Part model, mm, in its own coordinate system. A direction names the side the tool comes from. Round coordinates to 2 decimals unless told otherwise and drop trailing zeros. Order: outer loops, then holes, each group sorted by start corner. A loop starts at its lowest first (then second) coordinate and runs counter-clockwise, first axis right, second up. Notation, with made-up numbers: (45.5, 30.25) -> (96.5, 30.25) arc R19 cw to (96.5, 52.25) -> close; hole circle Ø5 at (10.25, 82). An arc over 180 degrees is marked (long way). Answer as a JSON object with one key per item and string values. Group by question number.
```python
from build123d import *

# Parameters (mm, degrees)
F1_DEPTH = 76.2
F3_DEPTH = 25.4
F4_DEPTH = 25.4
F5_DEPTH = 38.1
F6_DEPTH = 38.1
F7_DEPTH = 38.1
F8_DEPTH = 38.1
F9_DEPTH = 38.1


with BuildPart() as f1:
    # F0 (on Front) → F1 (new body)
    with BuildSketch(Plane.XZ):
        Polygon((22.4569932461, 74.4162100717), (-18.4116067539, 74.4162100717), (-26.8437221389, 1.1637246492), (13.1697589532, 0), align=None)
    extrude(amount=F1_DEPTH)

    # F2 (on Front) + F1_face (on face) → F3 (cut)
    with BuildSketch(Plane.XZ):
        Polygon((12.081772089, 66.8269023299), (-11.4912800491, 66.8269023299), (-18.7445282936, 10.2515770122), (4.1031986475, 10.2515770122), align=None)
    with BuildSketch(Plane(origin=(-2.3405186652, -76.2, 37.6069334432), x_dir=(1, 0, 0), z_dir=(0, -1, 0))):
        Polygon((-24.5032034737, -36.443208794), (15.5102776183, -37.6069334432), (24.7975119113, 36.8092766285), (-16.0710880887, 36.8092766285), align=None)
    extrude(amount=-F3_DEPTH, mode=Mode.SUBTRACT)

    # F2 (on Front) + F3_face (on face) → F4 (cut)
    with BuildSketch(Plane.XZ):
        Polygon((12.081772089, 66.8269023299), (-11.4912800491, 66.8269023299), (-18.7445282936, 10.2515770122), (4.1031986475, 10.2515770122), align=None)
    with BuildSketch(Plane(origin=(-2.3405186652, -50.8, 37.6069334432), x_dir=(1, 0, 0), z_dir=(0, -1, 0))):
        Polygon((-16.0710880887, 36.8092766285), (-24.5032034737, -36.443208794), (15.5102776183, -37.6069334432), (24.7975119113, 36.8092766285), align=None)
    extrude(amount=-F4_DEPTH, mode=Mode.SUBTRACT)

    # F2 (on Front) → F5 (cut, symmetric)
    with BuildSketch(Plane.XZ):
        Polygon((12.081772089, 66.8269023299), (-11.4912800491, 66.8269023299), (-18.7445282936, 10.2515770122), (4.1031986475, 10.2515770122), align=None)
    extrude(amount=F5_DEPTH, both=True, mode=Mode.SUBTRACT)

    # F2 (on Front) → F6 (join, symmetric)
    with BuildSketch(Plane.XZ):
        Polygon((12.081772089, 66.8269023299), (-11.4912800491, 66.8269023299), (-18.7445282936, 10.2515770122), (4.1031986475, 10.2515770122), align=None)
    extrude(amount=F6_DEPTH, both=True)

    # F7 (cut, symmetric): a face of the model
    f7_faces = [f1.faces().sort_by_distance(p)[0] for p in [
        (-3.4928762861, -38.1, 38.6865713538),
    ]]
    extrude(f7_faces, amount=F7_DEPTH, both=True, mode=Mode.SUBTRACT)

    # F8 (cut, symmetric): a face of the model
    f8_faces = [f1.faces().sort_by_distance(p)[0] for p in [
        (-3.4928762861, 38.1, 38.6865713538),
    ]]
    extrude(f8_faces, amount=F8_DEPTH, both=True, mode=Mode.SUBTRACT)

    # F2 (on Front) → F9 (cut, symmetric)
    with BuildSketch(Plane.XZ):
        Polygon((12.081772089, 66.8269023299), (-11.4912800491, 66.8269023299), (-18.7445282936, 10.2515770122), (4.1031986475, 10.2515770122), align=None)
    extrude(amount=F9_DEPTH, both=True, mode=Mode.SUBTRACT)


solid = f1.part
```
Q1. Band-saw the part on A-A (x = 10.5). List the corners of the cut face in (y, z).
Q2. Band-saw the part on D-D (x = -21). List the corners of the cut face in (y, z), plus the area to 3 significant figures.
Q3. Two-plate mould, pull along X, no slides. Class faces 3 (the flat face through (17.75, -12.52, 36.69)), 4 (the flat face through (8.4, 0, 37.7)), 5 (the flat face through (8.037, -12.878, 38.143)), 6 (the flat face through (-22.57, -12.52, 38.3)): +X half, -X half, draft (parallel to the pull), parting line (faces both ways), or undercut.
Q4. Band-saw the part on B-B (z = 26.5). List the corners of the cut face in (x, y).
Q5. Band-saw the part on C-C (y = -10.5). List the corners of the cut face in (x, z).
Q6. Wall check: line 1 (Z direction, x = 0, y = -16.5); line 2 (Z direction, x = -4, y = -3); line 3 (X direction, y = -20.25, z = 48.5). Give the ranges that are in metal, low to high. Write a range as [from, to].
Q7. Which spindle directions (+Z, -Z, +X, -X, +Y, -Y) get a long thin tool onto all of the face, cutting with end or side? Do faces 1 (the flat face through (8.4, -25.4, 37.7)), 2 (the flat face through (-7, -13, 10.252)). Say none if no direction does.
Q8. Drop flat-ended pins along their axis: pin 1 Ø12 at (x, y) = (-5, -18) entering from -Z; pin 2 Ø2 at (y, z) = (-2.5, 36.5) entering from -X; pin 3 Ø4 at (x, z) = (-20, 11.5) entering from +Y; pin 4 Ø4 at (y, z) = (-16, 38.5) entering from -X. Give the stop position or say it passes through.
Completed:
{
 "1": {"outline": "(-25.4, 0.08) -> (0, 0.08) -> (0, 55.61) -> (-25.4, 55.61) -> close; (-25.4, 66.83) -> (0, 66.83) -> (0, 74.42) -> (-25.4, 74.42) -> close"},
 "2": {"outline": "(-25.4, 0.99) -> (0, 0.99) -> (0, 51.93) -> (-25.4, 51.93) -> close", "area": "1,290 mm2"},
 "3": {"face 3": "+X half", "face 4": "draft", "face 5": "undercut", "face 6": "-X half"},
 "4": {"outline": "(-23.93, -25.4) -> (-16.66, -25.4) -> (-16.66, 0) -> (-23.93, 0) -> close; (6.39, -25.4) -> (16.48, -25.4) -> (16.48, 0) -> (6.39, 0) -> close"},
 "5": {"outline": "(-26.84, 1.16) -> (13.17, 0) -> (22.46, 74.42) -> (-18.41, 74.42) -> close; hole (-18.74, 10.25) -> (4.1, 10.25) -> (12.08, 66.83) -> (-11.49, 66.83) -> close"},
 "6": {"line 1": "[0.38, 10.25], [66.83, 74.42]", "line 2": "[0.5, 10.25], [66.83, 74.42]", "line 3": "[-21.39, -13.84], [9.5, 19.22]"},
 "7": {"face 1": "+Z, -Z, +X, -X, -Y", "face 2": "+Y, -Y"},
 "8": {"pin 1": "z = 0.35", "pin 2": "x = -22.89", "pin 3": "y = 0", "pin 4": "x = -22.78"}
}
